Check sheet for the modelled part. Datum: model origin and axes. Units: mm. A direction names the side the tool comes from. Coordinates: 2 decimals unless noted, no trailing zeros. Order: outer loops, then holes, each group sorted by start corner. A loop starts at its lowest first (then second) coordinate and runs counter-clockwise, first axis right, second up.
1. Gauge pin test, flat ends, axial feed: pin 1 Ø3 at (x, z) = (-10.5, -0.5) entering from +Y; pin 2 Ø2 at (y, z) = (24, -2.5) entering from +X; pin 3 Ø2 at (x, z) = (-10, 0) entering from +Y; pin 4 Ø3 at (y, z) = (26, -1.5) entering from -X. Record the tip position at first contact, or that the pin passes through.
2. Draft check along X on faces 1 (the cylindrical face through (20.5, 6, -0.1)), 2 (the cylindrical face through (-8.476, 7.098, 0.632)), 3 (the flat face through (5, 0, 0)), 4 (the cylindrical face through (28, 6, -5)). Enter one of: released by +X, released by -X, zero draft, split by the parting line, or undercut.
3. Thickness scan on line 1 (X direction, y = 5.5, z = 0); line 2 (X direction, y = 29, z = 0); line 3 (Y direction, x = 20, z = -0.5). Record the ranges inside material, lowest first.
4. Cross-section at B-B (z = 0). Count the separate pieces of the cut face and the enclosed holes in it, then the cut area to 3 significant figures.
5. Set-up check for faces 5 (the flat face through (19.2, 26, 5.5)), 6 (the flat face through (11.683, 23.881, -5.493)), 7 (the flat face through (20, 25.5, 0)): record each of +Z, -Z, +X, -X, +Y, -Y from which the full face is reachable in a straight line by a thin tool's end or side.
6. Cross-section at D-D (y = 17). Enter the section's corners in (x, z).
7. Cross-section at C-C (x = 23). Enter the section's corners in (y, z), then the cut area to 3 significant figures.
8. Cross-section at A-A (x = -10). Enter the section's corners in (y, z).
```python
from build123d import *

# Parameters (mm, degrees)
BOSS_EXTRUDE1_DEPTH = 6
SKETCH2_R           = 1.65
CUT_EXTRUDE1_DEPTH  = 20
SKETCH3_R           = 2.5
CUT_EXTRUDE2_DEPTH  = 30
CHAMFER1_SIZE       = 4
FILLET1_R           = 4
FILLET2_R           = 5
CHAMFER2_SIZE       = 1


with BuildPart() as part:
    # Sketch1 → Boss-Extrude1 (new body, symmetric)
    with BuildSketch(Plane.XY):
        Polygon((0, 14), (0, 34), (30, 34), (30, 25.5), (10, 25.5), (10, 11.8), (30, 11.8), (30, 0), (0, 0), (-20, 0), (-20, 14), align=None)
    extrude(amount=BOSS_EXTRUDE1_DEPTH, both=True)

    # Sketch2 → Cut-Extrude1 (cut)
    with BuildSketch(Plane(origin=(0, 14, 0), x_dir=(1, 0, 0), z_dir=(0, 1, 0))):
        with Locations((-10, 0)):
            Circle(SKETCH2_R)
    extrude(amount=-CUT_EXTRUDE1_DEPTH, mode=Mode.SUBTRACT)

    # Sketch3 → Cut-Extrude2 (cut, symmetric)
    with BuildSketch(Plane(origin=(0, 11.8, 0), x_dir=(1, 0, 0), z_dir=(0, 1, 0))):
        with Locations((23, 0)):
            Circle(SKETCH3_R)
    extrude(amount=CUT_EXTRUDE2_DEPTH, both=True, mode=Mode.SUBTRACT)

    # Chamfer1
    chamfer1_edges = [part.edges().sort_by_distance(p)[0] for p in [
        (0, 14, 0),
        (10, 25.5, 0),
        (10, 11.8, 0),
    ]]
    chamfer(chamfer1_edges, length=CHAMFER1_SIZE)

    # Fillet1
    fillet1_edges = [part.edges().sort_by_distance(p)[0] for p in [
        (0, 34, 0),
    ]]
    fillet(fillet1_edges, radius=FILLET1_R)

    # Fillet2
    fillet2_edges = [part.edges().sort_by_distance(p)[0] for p in [
        (-20, 7, -6),
        (30, 29.75, -6),
        (30, 5.9, 6),
        (30, 5.9, -6),
        (30, 29.75, 6),
        (-20, 7, 6),
    ]]
    fillet(fillet2_edges, radius=FILLET2_R)

    # Chamfer2
    chamfer2_edges = [part.edges().sort_by_distance(p)[0] for p in [
        (-9.5, 14, -6),
        (-9.5, 14, 6),
        (10, 18.65, -6),
        (10, 18.65, 6),
        (19.5, 25.5, -6),
        (19.5, 25.5, 6),
        (-2, 16, -6),
        (-2, 16, 6),
        (12, 13.8, -6),
        (12, 13.8, 6),
        (12, 23.5, -6),
        (12, 23.5, 6),
        (0, 24, -6),
        (0, 24, 6),
        (1.171572875, 32.828427125, -6),
        (1.171572875, 32.828427125, 6),
        (30, 34, 0),
        (30, 25.5, 0),
        (14.5, 34, -6),
        (14.5, 34, 6),
        (28.535533906, 34, 4.535533906),
        (28.535533906, 34, -4.535533906),
        (19.5, 11.8, -6),
        (5, 0, -6),
        (28.535533906, 25.5, 4.535533906),
        (28.535533906, 25.5, -4.535533906),
        (5, 0, 6),
        (19.5, 11.8, 6),
        (30, 11.8, 0),
        (30, 0, 0),
        (28.535533906, 11.8, 4.535533906),
        (28.535533906, 11.8, -4.535533906),
        (-20, 0, 0),
        (-18.535533906, 0, 4.535533906),
        (-18.535533906, 0, -4.535533906),
        (28.535533906, 0, 4.535533906),
        (28.535533906, 0, -4.535533906),
        (-20, 14, 0),
        (-18.535533906, 14, 4.535533906),
        (-18.535533906, 14, -4.535533906),
    ]]
    chamfer(chamfer2_edges, length=CHAMFER2_SIZE)


solid = part.part
```
Data:
1. pin 1: stops at y = 14
1. pin 2: stops at x = 13.5
1. pin 3: passes through
1. pin 4: stops at x = 0
2. face 1: undercut
2. face 2: undercut
2. face 3: zero draft
2. face 4: released by +X
3. line 1: x = -20 to -11.65, -8.35 to 20.5, 25.5 to 30
3. line 2: x = 0 to 20.5, 25.5 to 30
3. line 3: y = 0 to 11.8, 25.5 to 34
4. separate pieces: 4
4. enclosed holes: 0
4. area: 896 mm2
5. face 5: +Z, +X
5. face 6: -Z, +X
5. face 7: +Z, -Z, +X
6. outline: (-1, -5) - (0.41, -6) - (9, -6) - (10, -5) - (10, 5) - (9, 6) - (0.41, 6) - (-1, 5) - close
7. outline: (0, -5) - (1, -6) - (10.8, -6) - (11.8, -5) - (11.8, -2.5) - (0, -2.5) - close; (0, 2.5) - (11.8, 2.5) - (11.8, 5) - (10.8, 6) - (1, 6) - (0, 5) - close; (25.5, -5) - (26.5, -6) - (33, -6) - (34, -5) - (34, -2.5) - (25.5, -2.5) - close; (25.5, 2.5) - (34, 2.5) - (34, 5) - (33, 6) - (26.5, 6) - (25.5, 5) - close
7. area: 138 mm2
8. outline: (0, -5) - (1, -6) - (13, -6) - (14, -5) - (14, -1.65) - (0, -1.65) - close; (0, 1.65) - (14, 1.65) - (14, 5) - (13, 6) - (1, 6) - (0, 5) - close
